Here's how the part is built. I have some questions about the finished solid (model axes, mm). A direction names the side the tool comes from. Round coordinates to 2 decimals unless told otherwise and drop trailing zeros. Loops run counter-clockwise (first coordinate to the right, second up) from the corner with the lowest first, then second, coordinate; pieces in that order, holes last. Notation, with made-up numbers: M 52.5,52 L 62.5,52 A28 ccw 62.5,73 Z; hole C 51,-16.5 d1. An arc over 180 degrees is marked long. Put each result on its own line as item: value. Start each with the question number.
```python
from build123d import *

# Parameters (mm, degrees)
CHAMFER1_SIZE       = 0.5
CHAMFER1_SIZE2      = 1.866025404
CHAMFER2_SIZE       = 0.5
CHAMFER2_SIZE2      = 1.866025404
BOSS_EXTRUDE1_START = 7.4
BOSS_EXTRUDE1_DEPTH = 7.4


with BuildPart() as part:
    # Sketch2 → Revolve1 (revolve)
    with BuildSketch(Plane(origin=(0, 0, 0), x_dir=(0, 0, -1), z_dir=(1, 0, 0)), mode=Mode.PRIVATE) as revolve1_sk:
        Polygon((-16, 2.5), (-6.6, 2.5), (-6.6, 8.9), (-7.6, 8.9), (-7.6, 6.1), (-15, 6.1), (-15, 8.9), (-16, 8.9), align=None)
    revolve(revolve1_sk.sketch.rotate(Axis((0, 0, 79.609460318), (0, 0, -1)), 90), axis=Axis((0, 0, 79.609460318), (0, 0, -1)))

    # Chamfer1
    chamfer1_edges = [part.edges().sort_by_distance(p)[0] for p in [
        (-8.9, 0, 15),
    ]]
    chamfer1_side = [part.faces().sort_by_distance(p)[0] for p in [
        (-8.9, 0, 15.5),
    ]]
    chamfer(chamfer1_edges, length=CHAMFER1_SIZE, length2=CHAMFER1_SIZE2, reference=chamfer1_side[0])

    # Chamfer2
    chamfer2_edges = [part.edges().sort_by_distance(p)[0] for p in [
        (-8.9, 0, 7.6),
    ]]
    chamfer2_side = [part.faces().sort_by_distance(p)[0] for p in [
        (-8.9, 0, 7.1),
    ]]
    chamfer(chamfer2_edges, length=CHAMFER2_SIZE, length2=CHAMFER2_SIZE2, reference=chamfer2_side[0])

    # Sketch4 → Boss-Extrude1 (add)
    with BuildSketch(Plane.XY.offset(7.6).offset(BOSS_EXTRUDE1_START)):
        with BuildLine():
            Line((1.645655792, 5.873824735), (1.892869388, 6.634669948))
            Line((1.892869388, 6.634669948), (2.368397646, 6.48016145))
            Line((2.368397646, 6.48016145), (2.121184051, 5.719316237))
            ThreePointArc((2.121184051, 5.719316237), (1.885003666, 5.801444749), (1.645655792, 5.873824735))
        make_face()
        with BuildLine():
            Line((-0.25, 6.094874896), (-0.25, 6.894874896))
            Line((-0.25, 6.894874896), (0.25, 6.894874896))
            Line((0.25, 6.894874896), (0.25, 6.094874896))
            ThreePointArc((0.25, 6.094874896), (0, 6.1), (-0.25, 6.094874896))
        make_face()
        with BuildLine():
            Line((3.38022333, 5.077803683), (3.850451532, 5.725017278))
            Line((3.850451532, 5.725017278), (4.254960029, 5.431124652))
            Line((4.254960029, 5.431124652), (3.784731827, 4.783911057))
            ThreePointArc((3.784731827, 4.783911057), (3.585490039, 4.935003666), (3.38022333, 5.077803683))
        make_face()
        with BuildLine():
            Line((4.783911057, 3.784731827), (5.431124652, 4.254960029))
            Line((5.431124652, 4.254960029), (5.725017278, 3.850451532))
            Line((5.725017278, 3.850451532), (5.077803683, 3.38022333))
            ThreePointArc((5.077803683, 3.38022333), (4.935003666, 3.585490039), (4.783911057, 3.784731827))
        make_face()
        with BuildLine():
            Line((5.719316237, 2.121184051), (6.48016145, 2.368397646))
            Line((6.48016145, 2.368397646), (6.634669948, 1.892869388))
            Line((6.634669948, 1.892869388), (5.873824735, 1.645655792))
            ThreePointArc((5.873824735, 1.645655792), (5.801444749, 1.885003666), (5.719316237, 2.121184051))
        make_face()
        with BuildLine():
            Line((6.094874896, 0.25), (6.894874896, 0.25))
            Line((6.894874896, 0.25), (6.894874896, -0.25))
            Line((6.894874896, -0.25), (6.094874896, -0.25))
            ThreePointArc((6.094874896, -0.25), (6.1, 0), (6.094874896, 0.25))
        make_face()
        with BuildLine():
            Line((5.873824735, -1.645655792), (6.634669948, -1.892869388))
            Line((6.634669948, -1.892869388), (6.48016145, -2.368397646))
            Line((6.48016145, -2.368397646), (5.719316237, -2.121184051))
            ThreePointArc((5.719316237, -2.121184051), (5.801444749, -1.885003666), (5.873824735, -1.645655792))
        make_face()
        with BuildLine():
            Line((5.077803683, -3.38022333), (5.725017278, -3.850451532))
            Line((5.725017278, -3.850451532), (5.431124652, -4.254960029))
            Line((5.431124652, -4.254960029), (4.783911057, -3.784731827))
            ThreePointArc((4.783911057, -3.784731827), (4.935003666, -3.585490039), (5.077803683, -3.38022333))
        make_face()
        with BuildLine():
            Line((3.784731827, -4.783911057), (4.254960029, -5.431124652))
            Line((4.254960029, -5.431124652), (3.850451532, -5.725017278))
            Line((3.850451532, -5.725017278), (3.38022333, -5.077803683))
            ThreePointArc((3.38022333, -5.077803683), (3.585490039, -4.935003666), (3.784731827, -4.783911057))
        make_face()
        with BuildLine():
            Line((2.121184051, -5.719316237), (2.368397646, -6.48016145))
            Line((2.368397646, -6.48016145), (1.892869388, -6.634669948))
            Line((1.892869388, -6.634669948), (1.645655792, -5.873824735))
            ThreePointArc((1.645655792, -5.873824735), (1.885003666, -5.801444749), (2.121184051, -5.719316237))
        make_face()
        with BuildLine():
            Line((0.25, -6.094874896), (0.25, -6.894874896))
            Line((0.25, -6.894874896), (-0.25, -6.894874896))
            Line((-0.25, -6.894874896), (-0.25, -6.094874896))
            ThreePointArc((-0.25, -6.094874896), (0, -6.1), (0.25, -6.094874896))
        make_face()
        with BuildLine():
            Line((-1.645655792, -5.873824735), (-1.892869388, -6.634669948))
            Line((-1.892869388, -6.634669948), (-2.368397646, -6.48016145))
            Line((-2.368397646, -6.48016145), (-2.121184051, -5.719316237))
            ThreePointArc((-2.121184051, -5.719316237), (-1.885003666, -5.801444749), (-1.645655792, -5.873824735))
        make_face()
        with BuildLine():
            Line((-3.38022333, -5.077803683), (-3.850451532, -5.725017278))
            Line((-3.850451532, -5.725017278), (-4.254960029, -5.431124652))
            Line((-4.254960029, -5.431124652), (-3.784731827, -4.783911057))
            ThreePointArc((-3.784731827, -4.783911057), (-3.585490039, -4.935003666), (-3.38022333, -5.077803683))
        make_face()
        with BuildLine():
            Line((-4.783911057, -3.784731827), (-5.431124652, -4.254960029))
            Line((-5.431124652, -4.254960029), (-5.725017278, -3.850451532))
            Line((-5.725017278, -3.850451532), (-5.077803683, -3.38022333))
            ThreePointArc((-5.077803683, -3.38022333), (-4.935003666, -3.585490039), (-4.783911057, -3.784731827))
        make_face()
        with BuildLine():
            Line((-5.719316237, -2.121184051), (-6.48016145, -2.368397646))
            Line((-6.48016145, -2.368397646), (-6.634669948, -1.892869388))
            Line((-6.634669948, -1.892869388), (-5.873824735, -1.645655792))
            ThreePointArc((-5.873824735, -1.645655792), (-5.801444749, -1.885003666), (-5.719316237, -2.121184051))
        make_face()
        with BuildLine():
            Line((-6.094874896, -0.25), (-6.894874896, -0.25))
            Line((-6.894874896, -0.25), (-6.894874896, 0.25))
            Line((-6.894874896, 0.25), (-6.094874896, 0.25))
            ThreePointArc((-6.094874896, 0.25), (-6.1, 0), (-6.094874896, -0.25))
        make_face()
        with BuildLine():
            Line((-5.873824735, 1.645655792), (-6.634669948, 1.892869388))
            Line((-6.634669948, 1.892869388), (-6.48016145, 2.368397646))
            Line((-6.48016145, 2.368397646), (-5.719316237, 2.121184051))
            ThreePointArc((-5.719316237, 2.121184051), (-5.801444749, 1.885003666), (-5.873824735, 1.645655792))
        make_face()
        with BuildLine():
            Line((-5.077803683, 3.38022333), (-5.725017278, 3.850451532))
            Line((-5.725017278, 3.850451532), (-5.431124652, 4.254960029))
            Line((-5.431124652, 4.254960029), (-4.783911057, 3.784731827))
            ThreePointArc((-4.783911057, 3.784731827), (-4.935003666, 3.585490039), (-5.077803683, 3.38022333))
        make_face()
        with BuildLine():
            Line((-3.784731827, 4.783911057), (-4.254960029, 5.431124652))
            Line((-4.254960029, 5.431124652), (-3.850451532, 5.725017278))
            Line((-3.850451532, 5.725017278), (-3.38022333, 5.077803683))
            ThreePointArc((-3.38022333, 5.077803683), (-3.585490039, 4.935003666), (-3.784731827, 4.783911057))
        make_face()
        with BuildLine():
            Line((-2.121184051, 5.719316237), (-2.368397646, 6.48016145))
            Line((-2.368397646, 6.48016145), (-1.892869388, 6.634669948))
            Line((-1.892869388, 6.634669948), (-1.645655792, 5.873824735))
            ThreePointArc((-1.645655792, 5.873824735), (-1.885003666, 5.801444749), (-2.121184051, 5.719316237))
        make_face()
    extrude(amount=-BOSS_EXTRUDE1_DEPTH)


solid = part.part
```
1) I'm going to push flat-ended pins straight in: P1, Ø0.6, axis at x = 0, z = 10, coming from the -Y side; P2, Ø0.6, axis at x = 0, z = 11.5, coming from the +Y side; P3, Ø2, axis at y = 2.5, z = 12, coming from the +X side; P4, Ø4.5, axis at x = 0, y = 0, coming from the -Z side. Where does each tip first touch, or does it pass through?
2) Suppose I cut it at A-A (x = 0). Write out the boundary of the cut face in (y, z).
3) If I drill on probe 1 along Z at (x, y) = (-6.25, 3.25); probe 2 along X at (y, z) = (-4, 7.75); probe 3 along Y at (x, z) = (0, 9.75), over which ranges is the centre line in solid material (lowest first)? Write a range as from..to.
4) On a 3-axis mill with a long thin cutter (end or side, diameter ignored), from which of +Z, -Z, +X, -X, +Y, -Y can I reach the whole of each face in a straight line? I mean faces 5 (the face through (-0.964, 6.023, 11.352)), 6 (the face through (6.026, -0.944, 11.352)), 7 (the face through (2.76, 5.44, 11.35)). Say none if no direction works.
5) If we mould it in two halves opening along Z, with no side actions, what happens to faces 1 (the face through (-2, 2, 6.6)), 2 (the face through (0.964, -6.023, 11.352)), 3 (the face through (2, 2, 16)), 4 (the face through (-5.43, -2.78, 11.35))? For each: pulls with the +Z half, pulls with the -Z half, needs draft (parallel to the pull), parting line crosses it, or undercut.
Results are:
1. P1: y = -6.89
1. P2: y = 6.89
1. P3: x = 6.63
1. P4: through
2. outline: M -8.9,6.6 L -2.5,6.6 L -2.5,16 L -8.9,16 L -8.9,15.5 L -7.03,15 L -6.89,15 L -6.89,7.6 L -7.03,7.6 L -8.9,7.1 Z; M 2.5,6.6 L 8.9,6.6 L 8.9,7.1 L 7.03,7.6 L 6.89,7.6 L 6.89,15 L 7.03,15 L 8.9,15.5 L 8.9,16 L 2.5,16 Z
3. probe 1: 6.6..7.6, 15..16
3. probe 2: -5.62..-5.08, -4.61..4.61, 5.08..5.62
3. probe 3: -6.89..-2.5, 2.5..6.89
4. face 5: +Y
4. face 6: +X
4. face 7: none
5. face 1: pulls with the -Z half
5. face 2: undercut
5. face 3: pulls with the +Z half
5. face 4: undercut
